```python
from build123d import *

# Parameters (mm, degrees)
F1_DEPTH = 25


with BuildPart() as f1:
    # F0 (on Top) → F1 (new body)
    with BuildSketch(Plane.XY):
        with BuildLine():
            ThreePointArc((20.906867, 22.848913), (13.575228, 27.836723), (5.130714, 30.542523))
            ThreePointArc((5.130714, 30.542523), (-0.713577, 30.962247), (-6.532326, 30.273729))
            ThreePointArc((-6.532326, 30.273729), (-30.576246, 4.925761), (-15.709158, -26.690678))
            ThreePointArc((-15.709158, -26.690678), (-0.912134, -30.957034), (14.110414, -27.569297))
            ThreePointArc((14.110414, -27.569297), (26.421356, -16.158029), (30.970469, 0))
            ThreePointArc((30.970469, 0), (28.343125, 12.483478), (20.906867, 22.848913))
        make_face()
        Polygon((-7.467673, 2.424569), (-7.273707, 15.420259), (6.69181, 15.420259), (6.69181, 1.648707), (22.015087, 1.648707), (22.015087, -7.079741), (7.079741, -7.079741), (7.079741, -20.269398), (-7.855604, -20.269398), (-7.855604, -6.691811), (-24.148708, -6.691811), (-24.148708, 2.424569), align=None, mode=Mode.SUBTRACT)
        with BuildLine():
            ThreePointArc((-6.532326, 35.712912), (-0.337296, 34.727729), (5.130714, 37.801791))
            ThreePointArc((5.130714, 37.801791), (6.5142, 39.851303), (7.324579, 42.187501))
            ThreePointArc((7.324579, 42.187501), (7.472775, 43.148763), (7.522346, 44.120117))
            ThreePointArc((7.522346, 44.120117), (-6.917762, 52.308751), (-6.532326, 35.712912))
        make_face()
        with BuildLine():
            ThreePointArc((-6.532326, 30.273729), (-0.713577, 30.962247), (5.130714, 30.542523))
            Line((5.130714, 30.542523), (5.130714, 37.801791))
            ThreePointArc((5.130714, 37.801791), (-0.337296, 34.727729), (-6.532326, 35.712912))
            Line((-6.532326, 35.712912), (-6.532326, 30.273729))
        make_face()
        with BuildLine():
            ThreePointArc((14.110414, -27.569297), (-0.912134, -30.957034), (-15.709158, -26.690678))
            Line((-15.709158, -26.690678), (0, -68.954743))
            Line((0, -68.954743), (14.110414, -27.569297))
        make_face()
        with BuildLine():
            Line((5.130714, 37.801791), (5.130714, 30.542523))
            ThreePointArc((5.130714, 30.542523), (13.575228, 27.836723), (20.906867, 22.848913))
            Line((20.906867, 22.848913), (25.3125, 29.579744))
            Line((25.3125, 29.579744), (34.622848, 35.204742))
            Line((34.622848, 35.204742), (34.622848, 42.187501))
            Line((34.622848, 42.187501), (72.252154, 38.502157))
            Line((72.252154, 38.502157), (14.256467, 66.821128))
            Line((14.256467, 66.821128), (14.256467, 42.187501))
            Line((14.256467, 42.187501), (7.324579, 42.187501))
            ThreePointArc((7.324579, 42.187501), (6.5142, 39.851303), (5.130714, 37.801791))
        make_face()
    extrude(amount=F1_DEPTH)


solid = f1.part
```
Input: part model. Units: mm. Frame: model coordinates. A direction names the side the tool comes from. Give positions to 0.01 mm unless a question says otherwise; leave off trailing zeros. Loops run counter-clockwise (first coordinate to the right, second up) from the corner with the lowest first, then second, coordinate; pieces in that order, holes last.
1) Section query C-C on y = 10. Return the cut outline in (x, z).
A:
outline: (-29.31, 0) - (-7.35, 0) - (-7.35, 25) - (-29.31, 25) - close; (6.69, 0) - (29.31, 0) - (29.31, 25) - (6.69, 25) - close
2) Contact query for flat-ended pins moving along their axis: pin 1 (8 mm diameter, centred on y = 2.5, z = 12.5, fed in from +X); pin 2 (8 mm diameter, centred on x = 49, z = 16, fed in from +Y); pin 3 (4 mm diameter, centred on y = -14, z = 6.5, fed in from -X); pin 4 (5 mm diameter, centred on x = 13, y = -2, fed in from -Z). Output: stop coordinate, or through.
A:
pin 1: stops at x = 30.97
pin 2: stops at y = 51.81
pin 3: stops at x = -28.55
pin 4: passes through
3) Section query D-D on x = 58. Return the cut outline in (y, z).
A:
outline: (39.9, 0) - (45.46, 0) - (45.46, 25) - (39.9, 25) - close
4) Line query: L1, parallel to Y at x = 21, z = 7; L2, parallel to X at y = -10.5, z = 6.5; L3, parallel to X at y = -11, z = 2. Output: solid intervals per line, ascending.
A:
L1: y = -22.76 to -7.08, 1.65 to 22.76, 22.99 to 63.53
L2: x = -29.14 to -7.86, 7.08 to 29.14
L3: x = -28.95 to -7.86, 7.08 to 28.95
5) Section query A-A on z = 5.5. Return the cut outline in (x, y).
A:
outline: (-15.71, -26.69) - (0, -68.95) - (14.11, -27.57) arc R30.97 ccw to (30.97, 0) arc R30.97 ccw to (20.91, 22.85) - (25.31, 29.58) - (34.62, 35.2) - (34.62, 42.19) - (72.25, 38.5) - (14.26, 66.82) - (14.26, 42.19) - (7.32, 42.19) arc R9.54 ccw to (7.52, 44.12) arc R9.54 ccw (long way) to (-6.53, 35.71) - (-6.53, 30.27) arc R30.97 ccw to start; hole (-24.15, -6.69) - (-7.86, -6.69) - (-7.86, -20.27) - (7.08, -20.27) - (7.08, -7.08) - (22.02, -7.08) - (22.02, 1.65) - (6.69, 1.65) - (6.69, 15.42) - (-7.27, 15.42) - (-7.47, 2.42) - (-24.15, 2.42) - close
6) Reachability of faces 5 (the flat face through (29.9, 32.35, 12.32)), 6 (the flat face through (14.256, 55, 12)), 7 (the flat face through (-16, -6.692, 12)), 8 (the flat face through (-6.532, 33, 12)) from +Z, -Z, +X, -X, +Y, -Y: full face, straight path, thin tool, end or side. Return the list, or none.
A:
face 5: +Z, -Z, +X
face 6: +Z, -Z, +Y
face 7: +Z, -Z
face 8: +Z, -Z, -X
7) Section query B-B on y = 51. Return the cut outline in (x, z).
A:
outline: (-8.63, 0) - (4.59, 0) - (4.59, 25) - (-8.63, 25) - close; (14.26, 0) - (46.66, 0) - (46.66, 25) - (14.26, 25) - close
8) Mould query, pull axis X, two halves, no side actions, for faces 1 (the flat face through (11, 42.188, 12)), 2 (the flat face through (9, 4, 0)), 3 (the flat face through (34.623, 39, 12)), 4 (the flat face through (6.956, -48.552, 12.325)). Classes: released by +X, released by -X, zero draft, split by the parting line, or undercut.
A:
face 1: undercut
face 2: zero draft
face 3: undercut
face 4: released by +X
